from build123d import *

# Parameters (mm, degrees)
SKETCH2_W           = 120
SKETCH2_H           = 120
SKETCH2_R           = 2.5
SKETCH2_W_2         = 87.5
SKETCH2_H_2         = 87.5
BOSS_EXTRUDE1_DEPTH = 5
SKETCH3_W           = 95
SKETCH3_H           = 95
BOSS_EXTRUDE2_DEPTH = 95
CUT_EXTRUDE1_DEPTH  = 95
CUT_EXTRUDE4_REACH  = 191.621
SKETCH5_W           = 87.5
SKETCH5_H           = 87.5
CUT_EXTRUDE5_REACH  = 196.487
SKETCH9_W           = 87.5
SKETCH9_H           = 83.964466094
CUT_EXTRUDE7_DEPTH  = 87.5


with BuildPart() as part:
    # Sketch2 → Boss-Extrude1 (new body)
    with BuildSketch(Plane.XY):
        with Locations((60, -60)):
            Rectangle(SKETCH2_W, SKETCH2_H)
        with Locations((10, -10.00000061)):
            Circle(SKETCH2_R, mode=Mode.SUBTRACT)
        with Locations((110, -10)):
            Circle(SKETCH2_R, mode=Mode.SUBTRACT)
        with Locations((9.988952602, -110)):
            Circle(SKETCH2_R, mode=Mode.SUBTRACT)
        with Locations((109.988952602, -110)):
            Circle(SKETCH2_R, mode=Mode.SUBTRACT)
        with Locations((60, -60)):
            Rectangle(SKETCH2_W_2, SKETCH2_H_2, mode=Mode.SUBTRACT)
    extrude(amount=BOSS_EXTRUDE1_DEPTH)

    # Sketch3 → Boss-Extrude2 (add)
    with BuildSketch(Plane.XY.offset(5)):
        with Locations((60, -60)):
            Rectangle(SKETCH3_W, SKETCH3_H)
    extrude(amount=BOSS_EXTRUDE2_DEPTH)

    # Sketch4 → Cut-Extrude1 (cut)
    with BuildSketch(Plane(origin=(107.5, 0, 0), x_dir=(0, 0, -1), z_dir=(1, 0, 0))):
        Polygon((-5, -12.5), (-100, -107.5), (-100, -12.5), align=None)
    extrude(amount=-CUT_EXTRUDE1_DEPTH, mode=Mode.SUBTRACT)

    # Cut-Extrude4: up to this plane
    cut_extrude4_end = Plane(origin=(12.5, -14.267766953, 3.232233047), z_dir=(0, -0.7071067811865476, -0.7071067811865476))
    # Sketch5 → Cut-Extrude4 (cut, up to the surface)
    with BuildSketch(Plane.XZ.offset(107.5), mode=Mode.PRIVATE) as cut_extrude4_sk1:
        with Locations((60, 52.5)):
            Rectangle(SKETCH5_W, SKETCH5_H)
    cut_extrude4_tool1 = split(extrude(cut_extrude4_sk1.sketch, amount=-CUT_EXTRUDE4_REACH, mode=Mode.PRIVATE), bisect_by=cut_extrude4_end, keep=Keep.BOTH, mode=Mode.PRIVATE)
    add(cut_extrude4_tool1.solids().sort_by_distance((60, -107.5, 52.5))[0], mode=Mode.SUBTRACT)

    # Cut-Extrude5: up to this plane
    cut_extrude5_end = Plane(origin=(12.5, -14.267766953, 3.232233047), z_dir=(0, -0.7071067811865476, -0.7071067811865476))
    # Sketch9 → Cut-Extrude5 (cut, up to the surface)
    with BuildSketch(Plane(origin=(0, 0, 5), x_dir=(-1, 0, 0), z_dir=(0, 0, -1)), mode=Mode.PRIVATE) as cut_extrude5_sk1:
        with Locations((-60, -61.767766953)):
            Rectangle(SKETCH9_W, SKETCH9_H)
    cut_extrude5_tool1 = split(extrude(cut_extrude5_sk1.sketch, amount=-CUT_EXTRUDE5_REACH, mode=Mode.PRIVATE), bisect_by=cut_extrude5_end, keep=Keep.BOTH, mode=Mode.PRIVATE)
    add(cut_extrude5_tool1.solids().sort_by_distance((60, -61.767767, 5))[0], mode=Mode.SUBTRACT)

    # Sketch10 → Cut-Extrude7 (cut)
    with BuildSketch(Plane.ZY.offset(-103.75)):
        Polygon((8.75, -19.785533906), (5, -19.785533906), (5, -16.25), align=None)
    extrude(amount=CUT_EXTRUDE7_DEPTH, mode=Mode.SUBTRACT)


solid = part.part
Model file for the job. Use its own axes, mm. A direction names the side the tool comes from. Give positions to 0.01 mm unless a question says otherwise; leave off trailing zeros. Write each loop counter-clockwise with the first axis right and the second up, starting at its lowest first coordinate (ties: lowest second). Pieces come first, ordered by that corner, then holes. Notation, with made-up numbers: M 10,76 L 47,76 A24 ccw 47,109 Z; hole C 87.5,-35.75 d2. An arc over 180 degrees is marked long. One line per item, written item: value. Start each with the question number.
Q1. Saw through at D-D, the plane z = 88. Write the cut outline in (x, y), plus the area to 3 significant figures.
Q2. Drop flat-ended pins along their axis: pin 1 Ø4 at (x, z) = (21, 10) entering from +Y; pin 2 Ø1.1 at (x, y) = (56.5, -105) entering from +Z; pin 3 Ø3 at (x, y) = (26, -79) entering from +Z. Give the stop position or say it passes through.
Q3. Saw through at C-C, the plane x = 110. Write the cut outline in (y, z), plus the area to 3 significant figures.
Q4. 3-axis set-ups, long thin cutter, end or side, ignore diameter. For faces 1 (the flat face through (0, -61, 2)), 2 (the flat face through (56, -107.5, 98)), 3 (the flat face through (60.612, -17.993, 6.849)): which of +Z, -Z, +X, -X, +Y, -Y reach the whole face in a straight line?
Q5. Saw through at A-A, the plane x = 75.5. Write the cut outline in (y, z).
Q6. Saw through at B-B, the plane y = -10. Write the cut outline in (x, z).
Q7. Two-plate mould, pull along X, no slides. Class faces 4 (the flat face through (59, -106, 8.75)), 5 (the flat face through (112, -59, 0)), 6 (the flat face through (12.5, -71, 41)), 7 (the flat face through (61, -103.75, 4)): +X half, -X half, draft (parallel to the pull), parting line (faces both ways), or undercut.
Q8. Probe probe 1 along Y at (x, z) = (110, 3.05); probe 2 along X at (y, z) = (-66.5, 45); probe 3 along Z at (x, y) = (109, -22). List the from-to ranges inside material, lowest first. Write a range as [from, to].
Output values:
1. outline: M 12.5,-107.5 L 16.25,-107.5 L 16.25,-99.04 L 103.75,-99.04 L 103.75,-107.5 L 107.5,-107.5 L 107.5,-95.5 L 12.5,-95.5 Z
1. area: 399 mm²
2. pin 1: stops at y = -15.5
2. pin 2: stops at z = 98.05
2. pin 3: stops at z = 73
3. outline: M -120,0 L -112.5,0 L -112.5,5 L -120,5 Z; M -107.5,0 L -12.5,0 L -12.5,5 L -107.5,5 Z; M -7.5,0 L 0,0 L 0,5 L -7.5,5 Z
3. area: 550 mm²
4. face 1: +Z, -Z, -X, +Y, -Y
4. face 2: +Z, +X, -X, -Y
4. face 3: -Z
5. outline: M -120,0 L -103.75,0 L -103.75,8.75 L -107.5,8.75 L -107.5,5 L -120,5 Z; M -107.5,96.25 L -107.29,96.25 L -19.79,8.75 L -16.25,5 L -16.25,0 L 0,0 L 0,5 L -12.5,5 L -107.5,100 Z
6. outline: M 0,0 L 7.5,0 L 7.5,5 L 0,5 Z; M 12.5,0 L 107.5,0 L 107.5,5 L 12.5,5 Z; M 112.5,0 L 120,0 L 120,5 L 112.5,5 Z
7. face 4: undercut
7. face 5: draft
7. face 6: -X half
7. face 7: undercut
8. probe 1: y = [-120, -112.5], [-107.5, -12.5], [-7.5, 0]
8. probe 2: x = [12.5, 16.25], [103.75, 107.5]
8. probe 3: z = [0, 5]
